Check sheet for the modelled part. Datum: model origin and axes. Units: mm. A direction names the side the tool comes from. Give positions to 0.01 mm unless a question says otherwise; leave off trailing zeros. Write each loop counter-clockwise with the first axis right and the second up, starting at its lowest first coordinate (ties: lowest second). Pieces come first, ordered by that corner, then holes. Notation, with made-up numbers: (21.25, -3) -> (42.25, -3) arc R28 ccw to (42.25, 19) -> close; hole circle Ø7 at (-32, 33). An arc over 180 degrees is marked (long way). Answer as a JSON object with one key per item and string values.
from build123d import *

# Parameters (mm, degrees)
SKETCH1_W            = 36
SKETCH1_H            = 33.5
SKETCH1_R            = 1.4
SKETCH1_W_2          = 3
SKETCH1_H_2          = 21
SKETCH1_W_3          = 16
SKETCH1_H_3          = 3
BASE_DEPTH           = 4
F_1MM_EDGE_FILLETS_R = 1


with BuildPart() as part:
    # Sketch1 → Base (new body)
    with BuildSketch(Plane(origin=(0, 0, 0), x_dir=(1, 0, 0), z_dir=(0, 1, 0))):
        Rectangle(SKETCH1_W, SKETCH1_H)
        with Locations(Location((11, -9.75, 0), (0, 0, 270))):
            Circle(SKETCH1_R, mode=Mode.SUBTRACT)
        with Locations(Location((11, 9.75, 0), (0, 0, 270))):
            Circle(SKETCH1_R, mode=Mode.SUBTRACT)
        with Locations((-12.5, -2.25)):
            Rectangle(SKETCH1_W_2, SKETCH1_H_2, mode=Mode.SUBTRACT)
        with Locations((-2, 11.5)):
            Rectangle(SKETCH1_W_3, SKETCH1_H_3, mode=Mode.SUBTRACT)
    extrude(amount=BASE_DEPTH)

    # 1mm Edge Fillets
    f_1mm_edge_fillets_edges = [part.edges().sort_by_distance(p)[0] for p in [
        (0, 0, 16.75),
        (-18, 0, 0),
        (0, 0, -16.75),
        (18, 0, 0),
        (18, 2, 16.75),
        (-18, 2, 16.75),
        (-18, 2, -16.75),
        (18, 2, -16.75),
    ]]
    fillet(f_1mm_edge_fillets_edges, radius=F_1MM_EDGE_FILLETS_R)


solid = part.part
1. Sectioned sample at C-C, the plane x = 11. Enter the section's corners in (y, z), plus the area to 3 significant figures.
Determined:
{"outline": "(0, -15.75) arc R1 ccw to (1, -16.75) -> (4, -16.75) -> (4, -11.15) -> (0, -11.15) -> close; (0, -8.35) -> (4, -8.35) -> (4, 8.35) -> (0, 8.35) -> close; (0, 11.15) -> (4, 11.15) -> (4, 16.75) -> (1, 16.75) arc R1 ccw to (0, 15.75) -> close", "area": "111 mm^2"}
2. Sectioned sample at B-B, the plane z = 9.75. Enter the section's corners in (x, y).
Determined:
{"outline": "(-18, 1) arc R1 ccw to (-17, 0) -> (-14, 0) -> (-14, 4) -> (-18, 4) -> close; (-11, 0) -> (9.6, 0) -> (9.6, 4) -> (-11, 4) -> close; (12.4, 0) -> (17, 0) arc R1 ccw to (18, 1) -> (18, 4) -> (12.4, 4) -> close"}
3. Sectioned sample at D-D, the plane y = 3.15. Enter the section's corners in (x, z), plus the area to 3 significant figures.
Determined:
{"outline": "(-18, -15.75) arc R1 ccw to (-17, -16.75) -> (17, -16.75) arc R1 ccw to (18, -15.75) -> (18, 15.75) arc R1 ccw to (17, 16.75) -> (-17, 16.75) arc R1 ccw to (-18, 15.75) -> close; hole (-14, -8.25) -> (-11, -8.25) -> (-11, 12.75) -> (-14, 12.75) -> close; hole (-10, -13) -> (6, -13) -> (6, -10) -> (-10, -10) -> close; hole circle Ø2.8 at (11, -9.75); hole circle Ø2.8 at (11, 9.75)", "area": "1,080 mm^2"}
4. Go/stop test with a flat-tipped pin: P1, Ø3, axis at x = -2.5, z = -12.5, coming from the +Y side. Record where the tip stops, or that it passes through.
Determined:
{"P1": "y = 4"}
5. Scan lines: L1, parallel to X at y = 3, z = 9.75; L2, parallel to Z at x = 0, y = 2.45; L3, parallel to X at y = 1.3, z = -9.75. Record each from-to range of solid material in increasing order. Write a range as [from, to].
Determined:
{"L1": "[-18, -14], [-11, 9.6], [12.4, 18]", "L2": "[-16.75, -13], [-10, 16.75]", "L3": "[-18, 9.6], [12.4, 18]"}
6. Sectioned sample at A-A, the plane x = 5.5. Enter the section's corners in (y, z), plus the area to 3 significant figures.
Determined:
{"outline": "(0, -15.75) arc R1 ccw to (1, -16.75) -> (4, -16.75) -> (4, -13) -> (0, -13) -> close; (0, -10) -> (4, -10) -> (4, 16.75) -> (1, 16.75) arc R1 ccw to (0, 15.75) -> close", "area": "122 mm^2"}
7. Mould release check, pull along Z, two halves, no side actions. Record for faces 3 (the face through (-2, 2, -13)), 4 (the face through (0, 0, 0)), 5 (the face through (11.95, 1.97, 8.72)), 6 (the face through (-17.715, 2.521, -16.449)): released by +Z, released by -Z, zero draft, split by the parting line, or undercut.
Determined:
{"face 3": "undercut", "face 4": "zero draft", "face 5": "undercut", "face 6": "released by -Z"}
8. Access from +Z, -Z, +X, -X, +Y, -Y to the whole of each face (thin tool, end or side, straight path). Record for faces 1 (the face through (17.699, 2.521, -16.465)), 2 (the face through (-11, 2, 2)).
Determined:
{"face 1": "-Z, +X, +Y, -Y", "face 2": "+Y, -Y"}
